Work out the finished part from the listing and answer in its coordinate system (mm). Face numbers are marked on the shaded views. A direction names the side the tool comes from. Round coordinates to 2 decimals unless told otherwise and drop trailing zeros. Order: outer loops, then holes, each group sorted by start corner. A loop starts at its lowest first (then second) coordinate and runs counter-clockwise, first axis right, second up. Notation, with made-up numbers: (27, -21.75) - (78, -21.75) arc R23 cw to (78, 10.25) - close; hole circle Ø7 at (-12, 30.25). An arc over 180 degrees is marked (long way). Put each result on its own line as item: value.
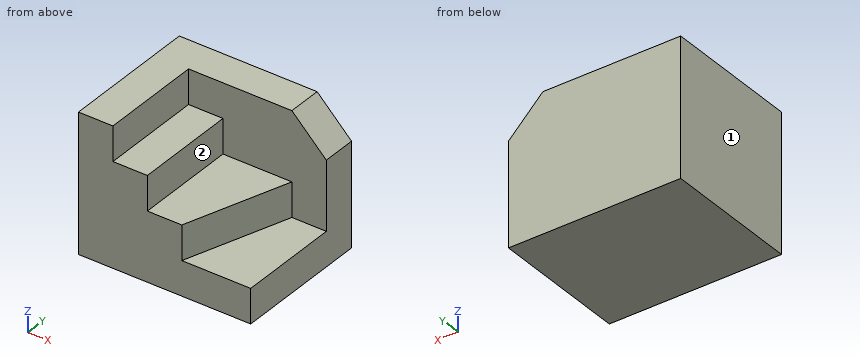
```python
from build123d import *

# Parameters (mm, degrees)
F1_DEPTH = 40
F0_W     = 10
F0_H     = 30
F2_DEPTH = 30
F3_DEPTH = 20
F4_DEPTH = 10
F5_SIZE  = 10


with BuildPart() as f1:
    # F0 (on Top) → F1 (new body)
    with BuildSketch(Plane.XY):
        Polygon((0, 40), (0, 0), (10, 0), (10, 30), (20, 30), (40, 30), (50, 30), (50, 40), align=None)
    extrude(amount=F1_DEPTH)

    # F0 (on Top) → F2 (join)
    with BuildSketch(Plane.XY):
        with Locations((15, 15)):
            Rectangle(F0_W, F0_H)
    extrude(amount=F2_DEPTH)

    # F0 (on Top) → F3 (join)
    with BuildSketch(Plane.XY):
        Polygon((20, 30), (20, 0), (30, 0), (40, 30), align=None)
    extrude(amount=F3_DEPTH)

    # F0 (on Top) → F4 (join)
    with BuildSketch(Plane.XY):
        Polygon((40, 30), (30, 0), (50, 0), (50, 30), align=None)
    extrude(amount=F4_DEPTH)

    # F5
    f5_edges = [f1.edges().sort_by_distance(p)[0] for p in [
        (50, 35, 40),
    ]]
    chamfer(f5_edges, length=F5_SIZE)


solid = f1.part
```
1) A cutting plane is placed at C-C on y = 22. Write down the section's boundary in (x, z).
Findings below:
outline: (0, 0) - (50, 0) - (50, 10) - (37.33, 10) - (37.33, 20) - (20, 20) - (20, 30) - (10, 30) - (10, 40) - (0, 40) - close
2) A cutting plane is placed at A-A on x = 13. Write down the section's boundary in (y, z), then the cut area to 3 significant figures.
Findings below:
outline: (0, 0) - (40, 0) - (40, 40) - (30, 40) - (30, 30) - (0, 30) - close
area: 1,300 mm2
3) Given pin 1 Ø10 at (x, y) = (42, 15.5) entering from +Z; pin 2 Ø3 at (y, z) = (18.5, 35) entering from +X; pin 3 Ø5 at (y, z) = (15, 27) entering from +X, each flat-ended and moving along its own axis, determine where each tip first touches the part or whether it passes through.
Findings below:
pin 1: stops at z = 10
pin 2: stops at x = 10
pin 3: stops at x = 20
4) For the marked faces 1 and 2, determine the directions among +Z, -Z, +X, -X, +Y, -Y from which every point of the face is accessible in a straight line to the end or side of a thin tool.
Findings below:
face 1: +Z, -Z, -X, +Y, -Y
face 2: +Z, +X, -Y
5) A cutting plane is placed at B-B on z = 36. Write down the section's boundary in (x, y), then the cut area to 3 significant figures.
Findings below:
outline: (0, 0) - (10, 0) - (10, 30) - (44, 30) - (44, 40) - (0, 40) - close
area: 740 mm2
6) Straight lines are drawn through the part: L1, parallel to Z at x = 39.5, y = 12; L2, parallel to Y at x = 25.5, z = 27; L3, parallel to Z at x = 24, y = 7.5. For each, find the intervals that lie inside material, in ascending order. Write a range as from..to.
Findings below:
L1: z = 0..10
L2: y = 30..40
L3: z = 0..20
7) A cutting plane is placed at D-D on x = 35.5. Write down the section's boundary in (y, z).
Findings below:
outline: (0, 0) - (40, 0) - (40, 40) - (30, 40) - (30, 20) - (16.5, 20) - (16.5, 10) - (0, 10) - close
